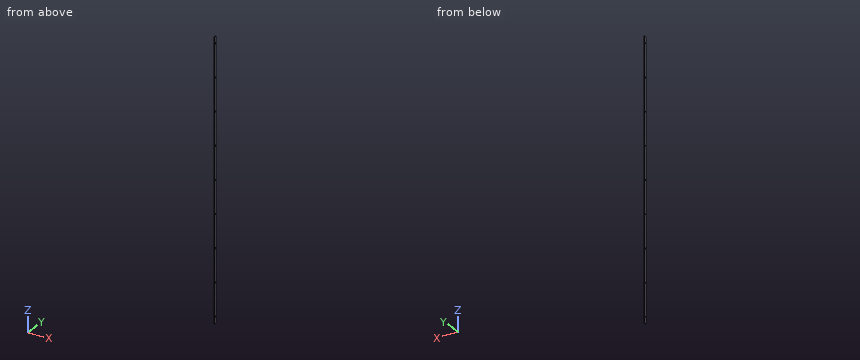
```python
from build123d import *

# Parameters (mm, degrees)
SKETCH1_W           = 1046
SKETCH1_H           = 8.541
BOSS_EXTRUDE1_DEPTH = 0.762
LPATTERN1_COUNT     = 9
LPATTERN1_PITCH     = 124.5
FILLET2_R           = 1


with BuildPart() as part:
    # Sketch1 → Boss-Extrude1 (new body)
    with BuildSketch(Plane(origin=(0, 0, 0), x_dir=(0, 0, -1), z_dir=(1, 0, 0))):
        Rectangle(SKETCH1_W, SKETCH1_H)
    extrude(amount=BOSS_EXTRUDE1_DEPTH)

    # Sketch2 → CSK for #2 Flat Head Machine Screw1 (revolve, cut)
    with BuildSketch(Plane(origin=(0.762, 0, 498), x_dir=(0, 0, -1), z_dir=(0, 1, 0))):
        Polygon((0, 0), (0, 0.762), (1.2192, 0.762), (1.2192, 1.110335587), (2.1844, 0), align=None)
    csk_for_2_flat_head_machine_screw1 = revolve(axis=Axis((7.112, 0, 498), (-1, 0, 0)), mode=Mode.SUBTRACT)

    # LPattern1: CSK for #2 Flat Head Machine Screw1 ×9
    with Locations(*[(0, 0, -i * LPATTERN1_PITCH) for i in range(1, LPATTERN1_COUNT)]):
        add(csk_for_2_flat_head_machine_screw1, mode=Mode.SUBTRACT)

    # Fillet2
    fillet2_edges = [part.edges().sort_by_distance(p)[0] for p in [
        (0.381, -4.2705, -523),
        (0.381, -4.2705, 523),
        (0.381, 4.2705, 523),
        (0.381, 4.2705, -523),
    ]]
    fillet(fillet2_edges, radius=FILLET2_R)


solid = part.part
```
Check sheet for the modelled part. Datum: model origin and axes. Units: mm. Coordinates: 2 decimals unless noted, no trailing zeros.
1) Sectioned sample at A-A (y = 0). Count the separate pieces of the cut face and the enclosed holes in it, and give its area (3 significant figures).
2) Material ranges on probe 1 along Z at (x, y) = (0.6, 3.75); probe 2 along Z at (x, y) = (0.55, 3.5); probe 3 along Y at (x, z) = (0.2, -372), recorded low to high.
3) Gauge pin test, flat end, axial feed: pin 1 (4 mm diameter, centred on y = -3, z = 376, fed in from -X). Record the tip position at first contact, or that the pin passes through.
Check sheet entries:
1. separate pieces: 10
1. enclosed holes: 0
1. area: 772 mm2
2. probe 1: z = -522.88 to 522.88
2. probe 2: z = -522.97 to 522.97
2. probe 3: y = -4.27 to -0.79, 0.79 to 4.27
3. pin 1: stops at x = 0
